```python
from build123d import *

# Parameters (mm, degrees)
F0_W     = 15.875
F0_H     = 25.273
F1_DEPTH = 1.524
F3_DEPTH = 0.762
F4_R     = 6.4135
F5_DEPTH = 17.526
F7_DEPTH = 25.4
F9_DEPTH = 25.4


with BuildPart() as f1:
    # F0 (on Top) → F1 (new body)
    with BuildSketch(Plane.XY):
        with BuildLine():
            Line((-7.9375, 13.6425291994), (-7.9375, 20.6375))
            Line((-7.9375, 20.6375), (-20.6375, 20.6375))
            Line((-20.6375, 20.6375), (-20.6375, 19.05))
            ThreePointArc((-20.6375, 19.05), (-18.931251337, 18.343248663), (-18.2245, 16.637))
            ThreePointArc((-18.2245, 16.637), (-18.931251337, 14.930751337), (-20.6375, 14.224))
            Line((-20.6375, 14.224), (-20.6375, 12.6365))
            Line((-20.6375, 12.6365), (-7.9375, 12.6365))
            Line((-7.9375, 12.6365), (-7.9375, 13.6425291994))
        make_face()
        with BuildLine():
            ThreePointArc((-7.9375, 13.6425291994), (-5.2899320117, 18.6392177438), (0, 20.6375))
            Line((0, 20.6375), (-7.9375, 20.6375))
            Line((-7.9375, 20.6375), (-7.9375, 13.6425291994))
        make_face()
        with BuildLine():
            ThreePointArc((7.9375, 13.6425291994), (5.2899320117, 18.6392177438), (0, 20.6375))
            ThreePointArc((0, 20.6375), (-5.2899320117, 18.6392177438), (-7.9375, 13.6425291994))
            Line((-7.9375, 13.6425291994), (-7.9375, 12.6365))
            Line((-7.9375, 12.6365), (7.9375, 12.6365))
            Line((7.9375, 12.6365), (7.9375, 13.6425291994))
        make_face()
        Rectangle(F0_W, F0_H)
        with BuildLine():
            Line((7.9375, -13.6425291994), (7.9375, -12.6365))
            Line((7.9375, -12.6365), (-7.9375, -12.6365))
            Line((-7.9375, -12.6365), (-7.9375, -13.6425291994))
            ThreePointArc((-7.9375, -13.6425291994), (-5.2899320117, -18.6392177438), (0, -20.6375))
            ThreePointArc((0, -20.6375), (5.2899320117, -18.6392177438), (7.9375, -13.6425291994))
        make_face()
        with BuildLine():
            Line((7.9375, -20.6375), (7.9375, -13.6425291994))
            ThreePointArc((7.9375, -13.6425291994), (5.2899320117, -18.6392177438), (0, -20.6375))
            Line((0, -20.6375), (7.9375, -20.6375))
        make_face()
        with BuildLine():
            Line((20.6375, -14.224), (20.6375, -12.6365))
            Line((20.6375, -12.6365), (7.9375, -12.6365))
            Line((7.9375, -12.6365), (7.9375, -13.6425291994))
            Line((7.9375, -13.6425291994), (7.9375, -20.6375))
            Line((7.9375, -20.6375), (20.6375, -20.6375))
            Line((20.6375, -20.6375), (20.6375, -19.05))
            ThreePointArc((20.6375, -19.05), (18.2245, -16.637), (20.6375, -14.224))
        make_face()
    extrude(amount=F1_DEPTH)

    # F2 (on face) → F3 (join)
    with BuildSketch(Plane.XY.offset(1.524)):
        with BuildLine():
            ThreePointArc((7.9375, 13.6425291994), (5.2899320117, 18.6392177438), (0, 20.6375))
            ThreePointArc((0, 20.6375), (-5.6575613563, 18.2940613563), (-8.001, 12.6365))
            Line((-8.001, 12.6365), (-7.9375, 12.6365))
            Line((-7.9375, 12.6365), (-7.9375, -13.6425291994))
            ThreePointArc((-7.9375, -13.6425291994), (-5.2899320117, -18.6392177438), (0, -20.6375))
            ThreePointArc((0, -20.6375), (5.6575613563, -18.2940613563), (8.001, -12.6365))
            Line((8.001, -12.6365), (7.9375, -12.6365))
            Line((7.9375, -12.6365), (7.9375, 13.6425291994))
        make_face()
    extrude(amount=F3_DEPTH)

    # F4 (on face) → F5 (join)
    with BuildSketch(Plane.XY.offset(2.286)):
        with BuildLine():
            ThreePointArc((-7.9375, -2.94e-08), (1.47e-08, -7.9375), (7.9375, 0))
            ThreePointArc((7.9375, 0), (-1.47e-08, 7.9375), (-7.9375, -2.94e-08))
        make_face()
        Circle(F4_R, mode=Mode.SUBTRACT)
    extrude(amount=F5_DEPTH)

    # F6 (on face) → F7 (cut)
    with BuildSketch(Plane.XY.offset(1.524)):
        with BuildLine():
            Line((-14.2875, 20.6375), (-20.6375, 20.6375))
            Line((-20.6375, 20.6375), (-20.6375, 19.05))
            ThreePointArc((-20.6375, 19.05), (-18.2245, 16.637), (-20.6375, 14.224))
            Line((-20.6375, 14.224), (-20.6375, 12.6365))
            Line((-20.6375, 12.6365), (-14.2875, 12.6365))
            Line((-14.2875, 12.6365), (-14.2875, 13.462))
            ThreePointArc((-14.2875, 13.462), (-17.4625, 16.637), (-14.2875, 19.812))
            Line((-14.2875, 19.812), (-14.2875, 20.6375))
        make_face()
        with BuildLine():
            Line((-14.2875, 13.462), (-14.2875, 19.812))
            ThreePointArc((-14.2875, 19.812), (-17.4625, 16.637), (-14.2875, 13.462))
        make_face()
        with BuildLine():
            ThreePointArc((-11.1125, 16.637), (-12.0424359697, 18.8820640303), (-14.2875, 19.812))
            Line((-14.2875, 19.812), (-14.2875, 13.462))
            ThreePointArc((-14.2875, 13.462), (-12.0424359697, 14.3919359697), (-11.1125, 16.637))
        make_face()
    extrude(amount=-F7_DEPTH, mode=Mode.SUBTRACT)

    # F8 (on face) → F9 (cut)
    with BuildSketch(Plane.XY.offset(1.524)):
        with BuildLine():
            ThreePointArc((14.2875, -13.462), (11.1125, -16.637), (14.2875, -19.812))
            Line((14.2875, -19.812), (14.2875, -13.462))
        make_face()
        with BuildLine():
            Line((14.2875, -13.462), (14.2875, -19.812))
            ThreePointArc((14.2875, -19.812), (16.5325640303, -18.8820640303), (17.4625, -16.637))
            ThreePointArc((17.4625, -16.637), (16.5325640303, -14.3919359697), (14.2875, -13.462))
        make_face()
        with BuildLine():
            Line((14.2875, -20.6375), (20.6375, -20.6375))
            Line((20.6375, -20.6375), (20.6375, -19.05))
            ThreePointArc((20.6375, -19.05), (18.2245, -16.637), (20.6375, -14.224))
            Line((20.6375, -14.224), (20.6375, -12.6365))
            Line((20.6375, -12.6365), (14.2875, -12.6365))
            Line((14.2875, -12.6365), (14.2875, -13.462))
            ThreePointArc((14.2875, -13.462), (16.5325640303, -14.3919359697), (17.4625, -16.637))
            ThreePointArc((17.4625, -16.637), (16.5325640303, -18.8820640303), (14.2875, -19.812))
            Line((14.2875, -19.812), (14.2875, -20.6375))
        make_face()
    extrude(amount=-F9_DEPTH, mode=Mode.SUBTRACT)


solid = f1.part
```
Here's how the part is built. I have some questions about the finished solid (model axes, mm). A direction names the side the tool comes from. Coordinates: 2 decimals unless noted, no trailing zeros. Order: outer loops, then holes, each group sorted by start corner. A loop starts at its lowest first (then second) coordinate and runs counter-clockwise, first axis right, second up.
Item 1: Which directions (+Z, -Z, +X, -X, +Y, -Y) give clear straight access to the entire face, cutting with the end or side of a thin tool? Please do faces 1 (the face through (6.117, 1.926, 10.926)), 2 (the face through (9, -17, 1.524)), 3 (the face through (7.938, 0, 1)), 4 (the face through (-7.938, 0, 1)), 5 (the face through (-9, 18, 1.524)).
Response values:
face 1: +Z
face 2: +Z, +X, -Y
face 3: +Z, -Z, +X, +Y
face 4: +Z, -Z, -X, -Y
face 5: +Z, -X, +Y
Item 2: If we section it at B-B, the plane y = 5: List the corners of the cut face in (x, z) for me, then the cut area to 3 significant figures.
Response values:
outline: (-7.94, 0) - (7.94, 0) - (7.94, 2.29) - (6.16, 2.29) - (6.16, 19.81) - (4.02, 19.81) - (4.02, 2.29) - (-4.02, 2.29) - (-4.02, 19.81) - (-6.16, 19.81) - (-6.16, 2.29) - (-7.94, 2.29) - close
area: 112 mm2
Item 3: If we section it at D-D, the plane x = -1: List the corners of the cut face in (y, z) for me, then the cut area to 3 significant figures.
Response values:
outline: (-20.57, 0) - (20.64, 0) - (20.64, 1.52) - (20.57, 1.52) - (20.57, 2.29) - (7.87, 2.29) - (7.87, 19.81) - (6.34, 19.81) - (6.34, 2.29) - (-6.34, 2.29) - (-6.34, 19.81) - (-7.87, 19.81) - (-7.87, 2.29) - (-20.57, 2.29) - close
area: 148 mm2
Item 4: If we section it at A-A, the plane x = 12.75: List the corners of the cut face in (y, z) for me.
Response values:
outline: (-20.64, 0) - (-19.41, 0) - (-19.41, 1.52) - (-20.64, 1.52) - close; (-13.86, 0) - (-12.64, 0) - (-12.64, 1.52) - (-13.86, 1.52) - close
Item 5: Thinking about a two-plate mould opening in Y: for faces 6 (the face through (11.113, -16.567, 0.773)), 7 (the face through (11, -12.636, 1)), 8 (the face through (-14.288, 20, 1)), which applies, pulls with the +Y half, pulls with the -Y half, needs draft (parallel to the pull), parting line crosses it, or undercut?
Response values:
face 6: undercut
face 7: pulls with the +Y half
face 8: needs draft
Item 6: I need wall thicknesses on probe 1 along Y at (x, z) = (0, 11.5); probe 2 along Z at (x, y) = (-5, 3.5); probe 3 along Y at (x, z) = (5, 9.75). Which ranges of each line are inside material? Lowest first, please.
Response values:
probe 1: y = -7.94 to -6.41, 6.41 to 7.94
probe 2: z = 0 to 2.29
probe 3: y = -6.16 to -4.02, 4.02 to 6.16
Item 7: I'm going to push flat-ended pins straight in: pin 1 Ø6 at (x, y) = (-4.5, -13) entering from +Z; pin 2 Ø8 at (x, y) = (1.5, -8.5) entering from +Z; pin 3 Ø1.8 at (y, z) = (-1.5, 1.5) entering from -X; pin 4 Ø3 at (y, z) = (-5.5, 16.5) entering from -X. Where does each tip first touch, or does it pass through?
Response values:
pin 1: stops at z = 2.29
pin 2: stops at z = 19.81
pin 3: stops at x = -7.94
pin 4: stops at x = -6.86
Item 8: If we section it at C-C, the plane z = 9.25: List the corners of the cut face in (x, y) for me (1 decimal).
Response values:
outline: circle Ø15.9 at (0, 0); hole circle Ø12.8 at (0, 0)
